Design review of the part built by this model. Coordinates are the model's own, in mm. A direction names the side the tool comes from. Give positions to 0.01 mm unless a question says otherwise; leave off trailing zeros. Write each loop counter-clockwise with the first axis right and the second up, starting at its lowest first coordinate (ties: lowest second). Pieces come first, ordered by that corner, then holes.
```python
from build123d import *

# Parameters (mm, degrees)
F0_W     = 10
F0_H     = 70
F1_DEPTH = 3.175


with BuildPart() as f1:
    # F0 (on Right) → F1 (new body)
    with BuildSketch(Plane.YZ):
        Polygon((36.825, -25), (26.825, 25), (-26.825, 25), (-36.825, -25), align=None)
        with Locations((31.825, 60)):
            Rectangle(F0_W, F0_H)
        Polygon((36.825, -25), (36.825, 25), (26.825, 25), align=None)
        Polygon((-36.825, -25), (-26.825, 25), (-36.825, 25), align=None)
        with Locations((-31.825, 60)):
            Rectangle(F0_W, F0_H)
    extrude(amount=F1_DEPTH)


solid = f1.part
```
(1) Consider section C-C, the plane y = 16. Give the boundary of the cut face in (x, z) (3 decimals), then the cut area to 3 significant figures.
Resolved:
outline: (0, -25) - (3.175, -25) - (3.175, 25) - (0, 25) - close
area: 159 mm2
(2) Tool access review of faces 4 (the face through (2, -26.825, 60)), 5 (the face through (2, -32, 95)): name each direction out of +Z, -Z, +X, -X, +Y, -Y from which nothing blocks a thin tool from reaching the whole face with its end or side.
Resolved:
face 4: +Z, +X, -X
face 5: +Z, +X, -X, +Y, -Y
(3) To check wall thickness, follow L1, parallel to Y at x = 2.75, z = 69.5 (3 decimals); L2, parallel to Z at x = 2.25, y = 6.5. State the ranges of each line that lie inside material, in increasing order.
Resolved:
L1: y = -36.825 to -26.825, 26.825 to 36.825
L2: z = -25 to 25
(4) Consider section B-B, the plane x = 2.6. Give the boundary of the cut face in (y, z) (3 decimals).
Resolved:
outline: (-36.825, -25) - (36.825, -25) - (36.825, 95) - (26.825, 95) - (26.825, 25) - (-26.825, 25) - (-26.825, 95) - (-36.825, 95) - close
(5) Mouldability with a two-part tool opening along Y and no side actions: class faces 1 (the face through (3.175, -1, 9)), 2 (the face through (2, 26.825, 60)), 3 (the face through (2, 36.825, 34)) as pulls with the +Y half, pulls with the -Y half, needs draft (parallel to the pull), parting line crosses it, or undercut.
Resolved:
face 1: needs draft
face 2: undercut
face 3: pulls with the +Y half
(6) Consider section A-A, the plane z = 64. Give the boundary of the cut face in (x, y) (3 decimals).
Resolved:
outline: (0, -36.825) - (3.175, -36.825) - (3.175, -26.825) - (0, -26.825) - close; (0, 26.825) - (3.175, 26.825) - (3.175, 36.825) - (0, 36.825) - close
(7) Clearance check with a flat-ended pin moving along its axis: P1, Ø1.6, axis at x = 1.5, y = -12, coming from the +Z side. State where the tip first meets the part, or that it passes through.
Resolved:
P1: stops at z = 25
